```python
from build123d import *

# Parameters (mm, degrees)
SKETCH1_R              = 10
BOSS_EXTRUDE1_DEPTH    = 3
FILLET1_R              = 0.5
SKETCH2_R              = 6
BOSS_EXTRUDE2_DEPTH    = 31
CHAMFER1_SIZE          = 0.5
SKETCH3_R              = 6
BOSS_EXTRUDE3_DEPTH    = 5
CUT_REVOLVE1_START     = -31
CUT_REVOLVE1_OUTLINE_W = 12
CUT_REVOLVE1_OUTLINE_H = 12
CUT_REVOLVE1_OUTLINE_R = 4
CUT_REVOLVE1_DEPTH     = 1.05
CHAMFER2_SIZE          = 1


# Read off the part's stored shape, not the designer's step: Cut-Revolve1
with BuildPart() as part:
    # Sketch1 → Boss-Extrude1 (new body)
    with BuildSketch(Plane.XY):
        Circle(SKETCH1_R)
    extrude(amount=BOSS_EXTRUDE1_DEPTH)

    # Fillet1
    fillet1_edges = [part.edges().sort_by_distance(p)[0] for p in [
        (-10, 0, 3),
    ]]
    fillet(fillet1_edges, radius=FILLET1_R)

    # Sketch2 → Boss-Extrude2 (add)
    with BuildSketch(Plane(origin=(0, 0, 0), x_dir=(-1, 0, 0), z_dir=(0, 0, -1))):
        Circle(SKETCH2_R)
    extrude(amount=BOSS_EXTRUDE2_DEPTH)

    # Chamfer1
    chamfer1_edges = [part.edges().sort_by_distance(p)[0] for p in [
        (6, 0, 0),
        (-10, 0, 0),
    ]]
    chamfer(chamfer1_edges, length=CHAMFER1_SIZE)

    # Sketch3 → Boss-Extrude3 (add)
    with BuildSketch(Plane(origin=(0, 0, -31), x_dir=(-1, 0, 0), z_dir=(0, 0, -1))):
        with Locations(Location((0, 0, 0), (0, 0, 180))):
            Circle(SKETCH3_R)
    extrude(amount=BOSS_EXTRUDE3_DEPTH)

    # Cut-Revolve1 outline → Cut-Revolve1 (cut)
    with BuildSketch(Plane.XY.offset(CUT_REVOLVE1_START)):
        Rectangle(CUT_REVOLVE1_OUTLINE_W, CUT_REVOLVE1_OUTLINE_H)
        Circle(CUT_REVOLVE1_OUTLINE_R, mode=Mode.SUBTRACT)
    extrude(amount=CUT_REVOLVE1_DEPTH, mode=Mode.SUBTRACT)

    # Chamfer2
    chamfer2_edges = [part.edges().sort_by_distance(p)[0] for p in [
        (-6, 0, -36),
    ]]
    chamfer(chamfer2_edges, length=CHAMFER2_SIZE)


solid = part.part
```
Input: part model. Units: mm. Frame: model coordinates. A direction names the side the tool comes from. Give positions to 0.01 mm unless a question says otherwise; leave off trailing zeros. Order: outer loops, then holes, each group sorted by start corner. A loop starts at its lowest first (then second) coordinate and runs counter-clockwise, first axis right, second up.
1. Section A-A on x = 0. Return the cut outline in (y, z), and give its area (3 significant figures).
Derived:
outline: (-10, 0.5) - (-9.5, 0) - (-6.5, 0) - (-6, -0.5) - (-6, -29.95) - (-4, -29.95) - (-4, -31) - (-6, -31) - (-6, -35) - (-5, -36) - (5, -36) - (6, -35) - (6, -31) - (4, -31) - (4, -29.95) - (6, -29.95) - (6, -0.5) - (6.5, 0) - (9.5, 0) - (10, 0.5) - (10, 2.5) arc R0.5 ccw to (9.5, 3) - (-9.5, 3) arc R0.5 ccw to (-10, 2.5) - close
area: 487 mm2
2. Section C-C on z = -24. Return the cut outline in (x, y).
Derived:
outline: circle Ø12 at (0, 0)
3. Mould query, pull axis Z, two halves, no side actions, for faces 1 (the flat face through (0, 0, -36)), 2 (the flat face through (-1.42, -3.92, -31)), 3 (the flat face through (0, 0, 3)), 4 (the cylindrical face through (5.723, -1.802, -32.972)). Classes: released by +Z, released by -Z, zero draft, split by the parting line, or undercut.
Derived:
face 1: released by -Z
face 2: undercut
face 3: released by +Z
face 4: zero draft
4. Material intervals for L1, parallel to Z at x = 1.75, y = -3.75; L2, parallel to Z at x = 7.25, y = 0; L3, parallel to X at y = -5.5, z = -24.5, sorted ascending.
Derived:
L1: z = -36 to -31, -29.95 to 3
L2: z = 0 to 3
L3: x = -2.4 to 2.4
5. Pin query (flat end, axial travel): pin 1 (12 mm diameter, centred on x = -4.5, z = -13.5, fed in from +Y); pin 2 (6 mm diameter, centred on y = 2.5, z = -12, fed in from -X); pin 3 (1.5 mm diameter, centred on y = -5.5, z = -8.5, fed in from -X). Return the tip coordinate at first contact, or that it passes through.
Derived:
pin 1: stops at y = 6
pin 2: stops at x = -6
pin 3: stops at x = -3.67
6. Reachability of faces 5 (the cylindrical face through (-0.867, -3.905, -30.482)), 6 (the cylindrical face through (-2.17, -9.76, 1.49)), 7 (the cylindrical face through (6, 0, -15)) from +Z, -Z, +X, -X, +Y, -Y: full face, straight path, thin tool, end or side. Return the list, or none.
Derived:
face 5: none
face 6: +Z, -Z
face 7: -Z
